Design review of the part built by this model. Coordinates are the model's own, in mm. A direction names the side the tool comes from. Coordinates: 2 decimals unless noted, no trailing zeros. Write each question's results on one line, items separated by ' | '. Start each with the question number.
```python
from build123d import *

# Parameters (mm, degrees)
F1_DEPTH = 40
F2_T     = -2.5
F3_W     = 10
F3_H     = 10
F4_DEPTH = 20
F5_W     = 10
F5_H     = 10
F6_DEPTH = 25
F7_R     = 4.99999
F8_R     = 2.49999


# Not quite as in the source:
# - a fillet or chamfer is up to 0.001 mm smaller than in the source, because OpenCascade refuses the exact size


with BuildPart() as f1:
    # F0 (on Top) → F1 (new body)
    with BuildSketch(Plane.XY):
        with BuildLine():
            Line((40.6640707215, 25), (0, 25))
            ThreePointArc((0, 25), (-25, 0), (0, -25))
            Line((0, -25), (40.6640707215, -25))
            Line((40.6640707215, -25), (40.6640707215, 25))
        make_face()
    extrude(amount=F1_DEPTH)

    # F2
    f2_openings = [f1.faces().sort_by_distance(p)[0] for p in [
        (10.256385, 0, 40),
    ]]
    offset(amount=F2_T, openings=f2_openings)

    # F3 (on face) → F4 (join)
    with BuildSketch(Plane.YZ.offset(40.6640707215)):
        with Locations((0, 5.0200799115)):
            Rectangle(F3_W, F3_H)
    extrude(amount=F4_DEPTH)

    # F5 (on face) → F6 (join)
    with BuildSketch(Plane.XY.offset(10.0200799115)):
        with Locations((55.6640707215, 0)):
            Rectangle(F5_W, F5_H)
    extrude(amount=F6_DEPTH)

    # F7 (radius 5 in the source; OpenCascade refuses exactly that, so slightly less here)
    f7_edges = [f1.edges().sort_by_distance(p)[0] for p in [
        (45.664071, -5, 10.02008),
        (45.664071, 5, 10.02008),
        (50.664071, -5, 22.52008),
        (50.664071, 5, 22.52008),
        (55.664071, -5, 35.02008),
        (60.664071, 0, 35.02008),
        (55.664071, 5, 35.02008),
        (50.664071, 0, 35.02008),
        (60.664071, -5, 17.52008),
        (60.664071, 5, 17.52008),
    ]]
    fillet(f7_edges, radius=F7_R)

    # F8 (radius 2.5 in the source; OpenCascade refuses exactly that, so slightly less here)
    f8_edges = [f1.edges().sort_by_distance(p)[0] for p in [
        (-22.5, 0, 40),
    ]]
    fillet(f8_edges, radius=F8_R)


solid = f1.part
```
Item 1: Insertion check: pin 1 Ø1.5 at (y, z) = (19, 4.5) entering from -X; pin 2 Ø1.5 at (y, z) = (11, 17.5) entering from +X; pin 3 Ø1.5 at (x, z) = (-4.5, 25.5) entering from +Y. Each pin has a flat end and moves straight along its axis. Give the tip position at first contact, or say it passes through.
Item 2: Wall thickness on L1, parallel to Y at x = 24.5, z = 31; L2, parallel to X at y = 0, z = 19.5; L3, parallel to X at y = 1, z = 33.5: over which ranges is each line inside the solid? List them lowest first.
Item 3: We need section A-A on z = 16.5. Count the separate pieces of the cut face and the enclosed holes in it, then the cut area to 3 significant figures.
Item 4: For faces 5 (the flat face through (48, -5, 3)), 6 (the cylindrical face through (52.09, -3.496, 20.473)), 7 (the flat face through (7, 0, 0)), 8 (the cylindrical face through (19, 23, 39)), 9 (the flat face through (48, 5, 3)), list the 3-axis set-ups (+Z, -Z, +X, -X, +Y, -Y) from which the entire face can be reached by the end or side of a thin tool; tool diameter is ignored.
Item 5: Draft analysis for pull direction X (two halves, no side actions). For faces 1 (the flat face through (20, -25, 20)), 2 (the cylindrical face through (46.6, 3.5, 8.59)), 3 (the flat face through (19, 22.5, 20)), 4 (the cylindrical face through (59.238, 3.496, 14.81)), state which applies: released by +X, released by -X, zero draft, split by the parting line, or undercut.
Answer:
1) pin 1: stops at x = -17.09 | pin 2: stops at x = 40.66 | pin 3: stops at y = 24.72
2) L1: y = -25 to -22.5, 22.5 to 25 | L2: x = -25 to -22.5, 38.16 to 40.66, 50.66 to 60.66 | L3: x = -24.98 to -22.48, 38.16 to 40.66, 52.22 to 59.11
3) separate pieces: 2 | enclosed holes: 1 | area: 581 mm^2
4) face 5: +Z, -Z, +X, -Y | face 6: +Z, -Y | face 7: -Z, +X, -X, +Y, -Y | face 8: +Z | face 9: +Z, -Z, +X, +Y
5) face 1: zero draft | face 2: undercut | face 3: undercut | face 4: released by +X
